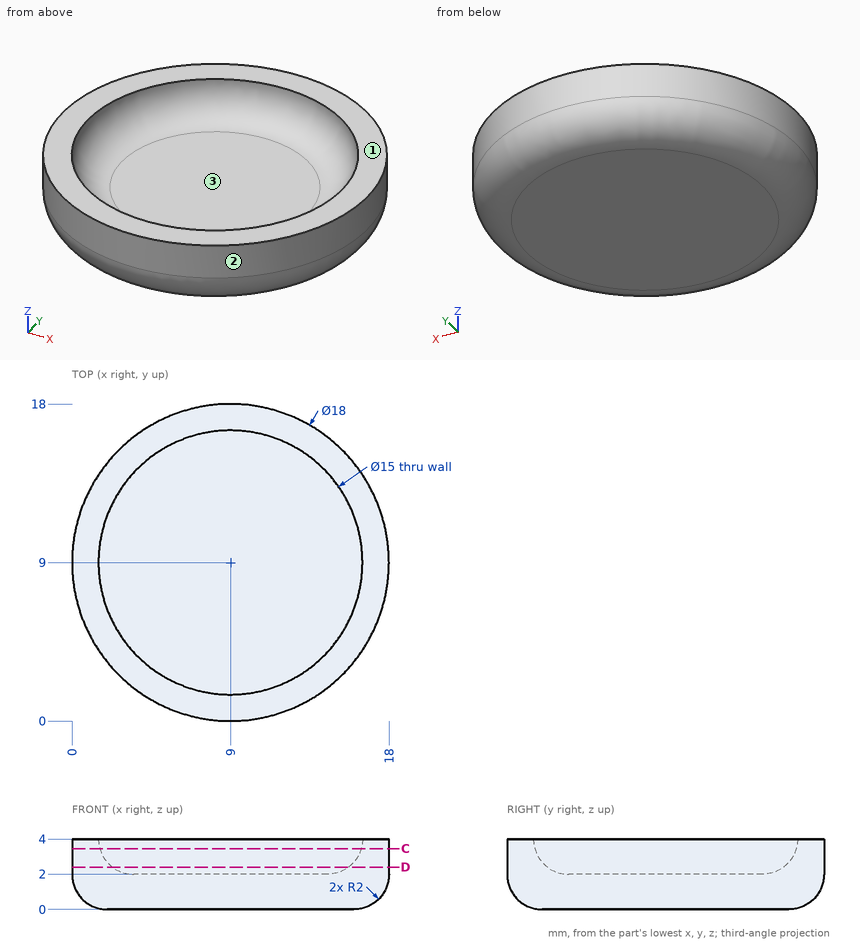
Geometry check sheet. Reference: drawing and pictorial views, mm from the part's lowest x, y, z. Coordinates: 2 decimals unless noted, no trailing zeros. Write each loop counter-clockwise with the first axis right and the second up, starting at its lowest first coordinate (ties: lowest second). Pieces come first, ordered by that corner, then holes. Notation, with made-up numbers: M 0,36 L 25,36 A12 cw 25,53 Z; hole C 28.25,-6.75 d10. An arc over 180 degrees is marked long. One line per question, with ' | ' between items.
1) Sectioned sample at C-C on z = 3.45. Record the cut outline in (x, y).
Solutions:
outline: C 9,9 d18; hole C 9,9 d14.85
2) Sectioned sample at D-D on z = 2.4. Record the cut outline in (x, y).
Solutions:
outline: C 9,9 d18; hole C 9,9 d13.4
3) Material ranges on L1, parallel to X at y = 5.25, z = 3.55; L2, parallel to X at y = 7.75, z = 2.95; L3, parallel to Z at x = 10, y = 11.75, recorded low to high.
Solutions:
L1: 0.82 to 2.56, 15.44 to 17.18 | L2: 0.09 to 1.91, 16.09 to 17.91 | L3: 0 to 2
4) Depth check by flat-ended pin: pin 1 Ø2 at (y, z) = (10.5, 0.5) entering from +X (3 decimals); pin 2 Ø1.5 at (y, z) = (6, 2.5) entering from +X. Enter the tip coordinate at first touch or a pass-through.
Solutions:
pin 1: x = 17.845 | pin 2: x = 17.71
5) Release check for a two-part mould opening along Y. For the marked faces 1, 2 and 3 record: +Y half, -Y half, draft (parallel to the pull), parting line (faces both ways), or undercut.
Solutions:
face 1: draft | face 2: parting line | face 3: undercut
